Could you check a few things on this drawing? It's one solid part, dimensions in mm from its lowest x, y, z. Give positions to 0.01 mm unless a question says otherwise; leave off trailing zeros. Write each loop counter-clockwise with the first axis right and the second up, starting at its lowest first coordinate (ties: lowest second). Pieces come first, ordered by that corner, then holes. Notation, with made-up numbers: M 55,2 L 68,2 A21 cw 68,8 Z; hole C 83.5,19 d4. An arc over 180 degrees is marked long. Use CSV: the item, a comma, the result in double quotes. Start each with the question number.
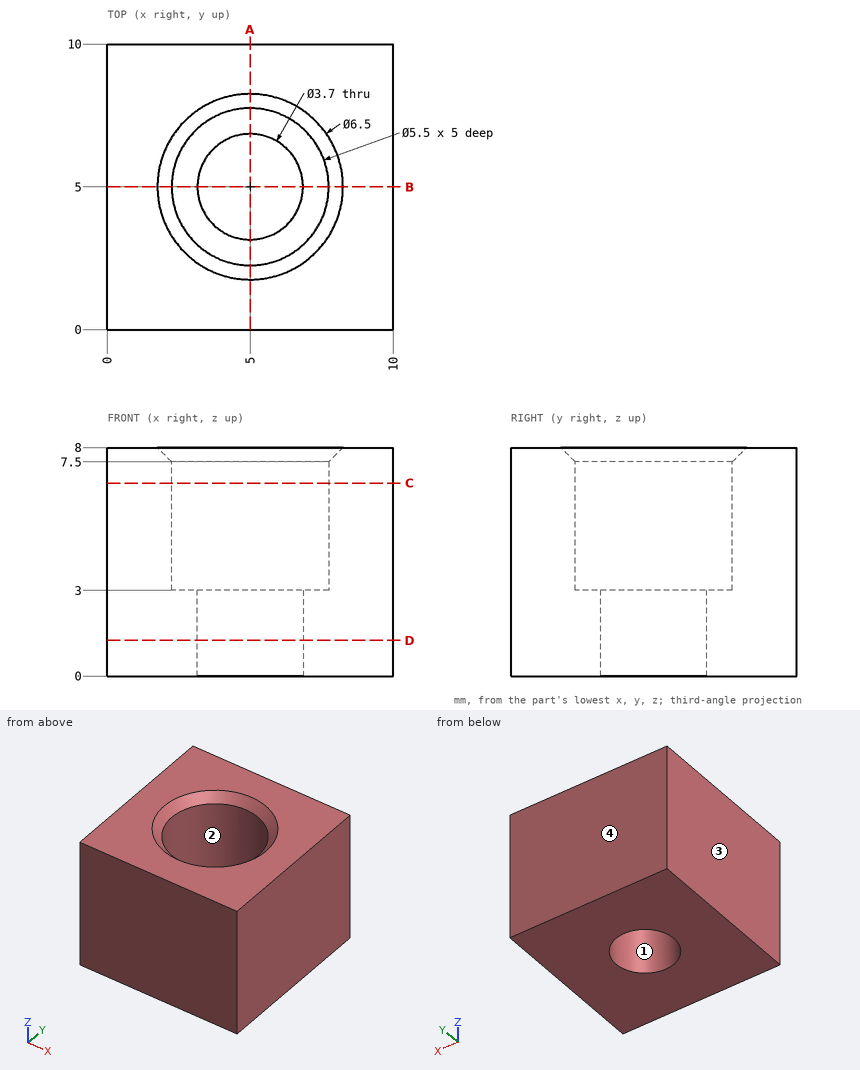
(1) Thinking about a two-plate mould opening in X: for the marked faces 1, 2, 3 and 4, which applies, released by +X, released by -X, zero draft, split by the parting line, or undercut?
(2) I want a section at D-D (z = 1.25). Write out the boundary of the cut face in (x, y), and give its area (3 significant figures).
(3) Will this pin go through, and if not, where does the flat tip stop? pin 1 Ø1.6 at (x, y) = (6, 6) entering from +Z.
(4) Please list where these lines run through material, in increasing order: L1, parallel to Y at x = 5, z = 5.1; L2, parallel to Y at x = 5, z = 1.4; L3, parallel to X at y = 6.25, z = 4. Write a range as [from, to].
(5) I want a section at A-A (x = 5). Write out the boundary of the cut face in (y, z), and give its area (4 significant figures).
(6) I want a section at C-C (z = 6.75). Write out the boundary of the cut face in (x, y).
Geometry results:
1,face 1,"undercut"
1,face 2,"undercut"
1,face 3,"released by -X"
1,face 4,"zero draft"
2,outline,"M 0,0 L 10,0 L 10,10 L 0,10 Z; hole C 5,5 d3.7"
2,area,"89.2 mm2"
3,pin 1,"stops at z = 3"
4,L1,"y = [0, 2.25], [7.75, 10]"
4,L2,"y = [0, 3.15], [6.85, 10]"
4,L3,"x = [0, 2.55], [7.45, 10]"
5,outline,"M 0,0 L 3.15,0 L 3.15,3 L 2.25,3 L 2.25,7.5 L 1.75,8 L 0,8 Z; M 6.85,0 L 10,0 L 10,8 L 8.25,8 L 7.75,7.5 L 7.75,3 L 6.85,3 Z"
5,area,"41.15 mm2"
6,outline,"M 0,0 L 10,0 L 10,10 L 0,10 Z; hole C 5,5 d5.5"
